Part print with two shaded views. Sizes in mm from the minimum x, y, z corner. A direction names the side the tool comes from. Give positions to 0.01 mm unless a question says otherwise; leave off trailing zeros. Write each loop counter-clockwise with the first axis right and the second up, starting at its lowest first coordinate (ties: lowest second). Pieces come first, ordered by that corner, then holes. Notation, with made-up numbers: M 12.5,59.5 L 27.5,59.5 A23 cw 27.5,75.5 Z; hole C 52,37 d4. An arc over 180 degrees is marked long. Return JSON: item names as keys, results as strings. Group by question number.
Q1. Pull direction X, two halves, no side cores. Call the marked faces 1, 2, 3 and 4: +X half, -X half, draft (parallel to the pull), parting line (faces both ways), or undercut.
Q2. Band-saw the part on A-A, the plane z = 9.5. Give the cut face in (x, y).
Q3. Band-saw the part on B-B, the plane y = 0.55. Give the cut face in (x, z), then the cut area to 3 significant figures.
Q4. Band-saw the part on D-D, the plane y = 2. Give the cut face in (x, z), then the cut area to 3 significant figures.
Q5. Flat gauge pins, fed straight in: pin 1 Ø0.8 at (x, y) = (8, 3) entering from -Z; pin 2 Ø1 at (y, z) = (2, 1) entering from +X; pin 3 Ø2 at (x, z) = (9.5, 19.5) entering from -Y; pin 4 Ø9 at (x, z) = (8.5, 7) entering from +Y. Where does each tip first touch, or does it go through?
Q6. Wall check: probe 1 along X at (y, z) = (0.7, 8); probe 2 along X at (y, z) = (1.5, 12.75); probe 3 along Z at (x, y) = (6.75, 0.65). Give the ranges that are in metal, low to high.
Q7. Band-saw the part on C-C, the plane x = 8. Give the cut face in (y, z).
Q8. Tool access for the marked faces 5, 6 and 7: list every direction of +Z, -Z, +X, -X, +Y, -Y with a clear straight run to the whole face (end or side of a thin tool).
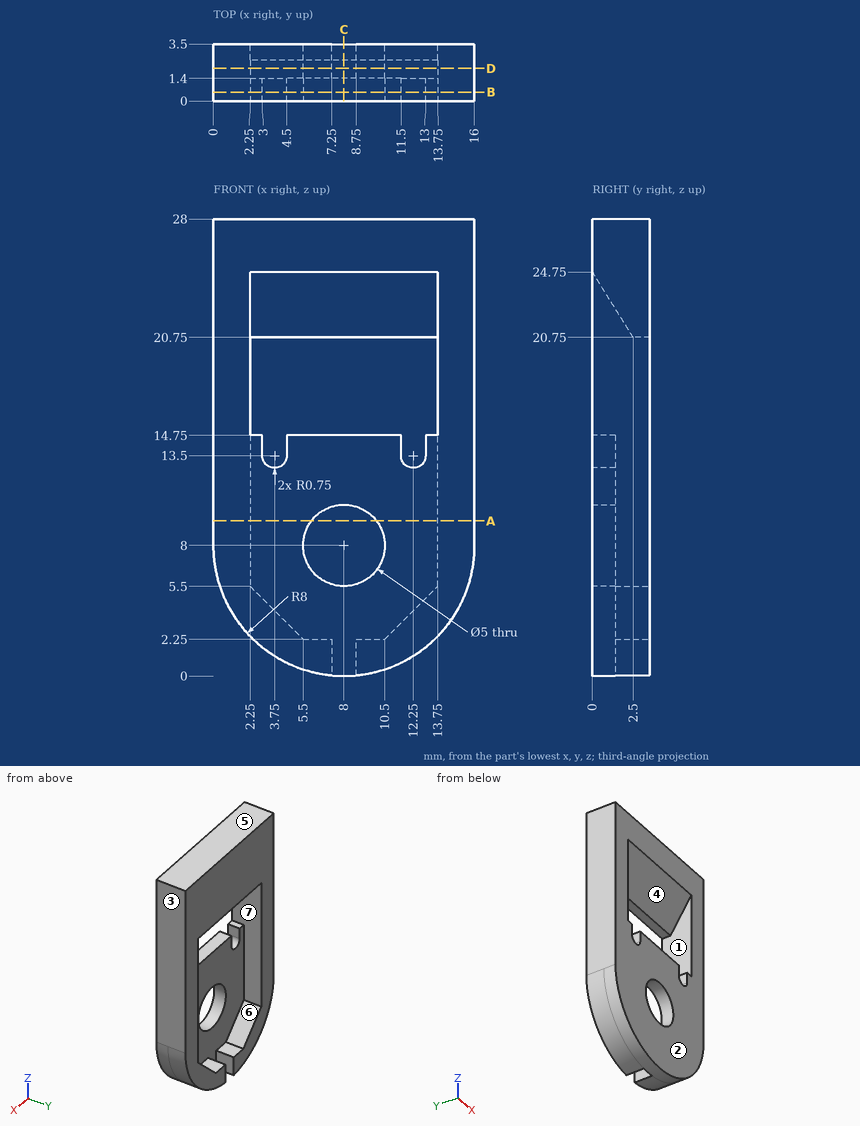
From the geometry:
{
 "1": {"face 1": "undercut", "face 2": "draft", "face 3": "+X half", "face 4": "undercut"},
 "2": {"outline": "M 0,0 L 6,0 L 6,1.4 L 2.25,1.4 L 2.25,3.5 L 0,3.5 Z; M 10,0 L 16,0 L 16,3.5 L 13.75,3.5 L 13.75,1.4 L 10,1.4 Z"},
 "3": {"outline": "M 0,8 A8 ccw 16,8 L 16,28 L 0,28 Z; hole M 2.25,14.75 L 3,14.75 L 3,13.5 A0.75 ccw 4.5,13.5 L 4.5,14.75 L 11.5,14.75 L 11.5,13.5 A0.75 ccw 13,13.5 L 13,14.75 L 13.75,14.75 L 13.75,23.87 L 2.25,23.87 Z; hole C 8,8 d5", "area": "290 mm^2"},
 "4": {"outline": "M 0,8 A8 ccw 7.25,0.04 L 7.25,2.25 L 5.5,2.25 L 2.25,5.5 L 2.25,21.55 L 13.75,21.55 L 13.75,5.5 L 10.5,2.25 L 8.75,2.25 L 8.75,0.04 A8 ccw 16,8 L 16,28 L 0,28 Z", "area": "206 mm^2"},
 "5": {"pin 1": "stops at z = 20.75", "pin 2": "stops at x = 12.66", "pin 3": "passes through", "pin 4": "stops at y = 1.4"},
 "6": {"probe 1": "x = 0 to 5.5, 10.5 to 16", "probe 2": "x = 0 to 2.25, 13.75 to 16", "probe 3": "z = 0.1 to 5.83, 10.17 to 14.75, 23.71 to 28"},
 "7": {"outline": "M 0,0 L 1.4,0 L 1.4,5.5 L 0,5.5 Z; M 0,10.5 L 1.4,10.5 L 1.4,14.75 L 0,14.75 Z; M 0,24.75 L 2.5,20.75 L 3.5,20.75 L 3.5,28 L 0,28 Z"},
 "8": {"face 5": "+Z, +X, -X, +Y, -Y", "face 6": "+Y", "face 7": "none"}
}
